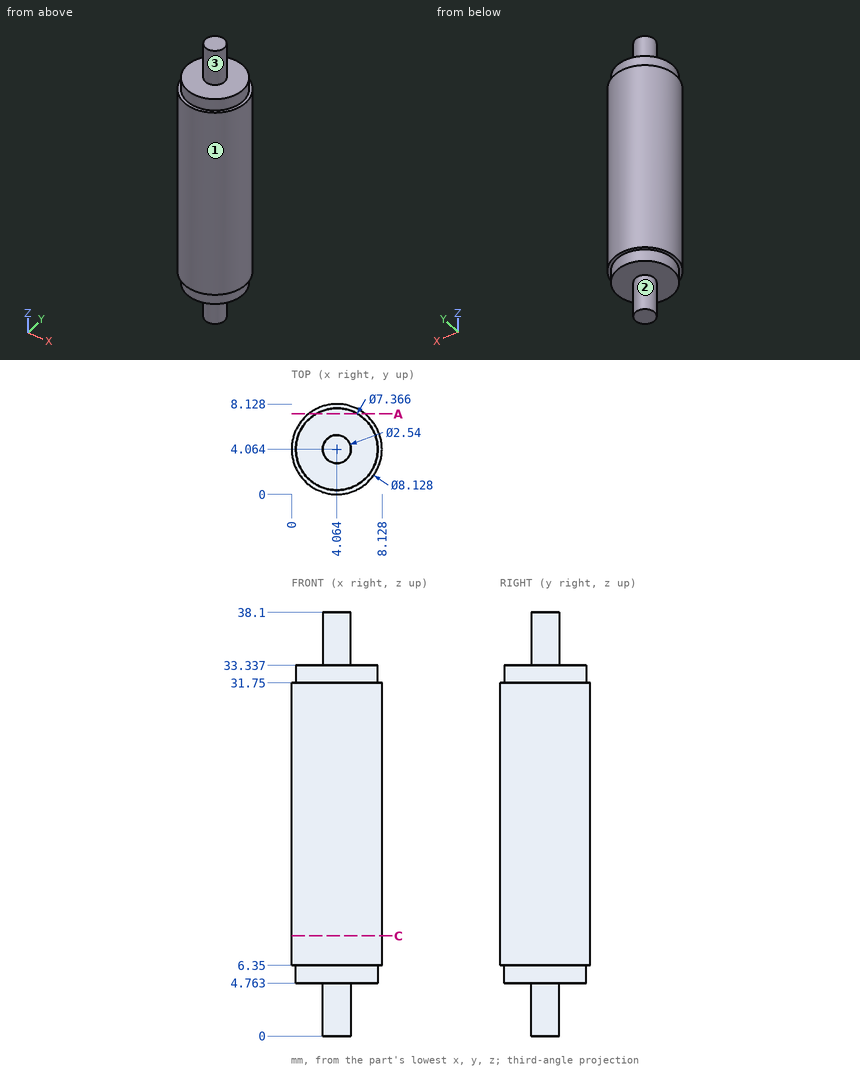
Input: dimensioned drawing with shaded views. Units: mm. Origin: part minimum x, y, z. A direction names the side the tool comes from. Give positions to 0.01 mm unless a question says otherwise; leave off trailing zeros. Order: outer loops, then holes, each group sorted by start corner. A loop starts at its lowest first (then second) coordinate and runs counter-clockwise, first axis right, second up.
(1) Access query for the marked faces 1, 2 and 3. Directions: +Z, -Z, +X, -X, +Y, -Y. A direction counts if a zero-diameter tool reaches every point of the face in a straight line with its end or side. Return the directions, or none.
(2) Contact query for flat-ended pins moving along their axis: P1, Ø1.5, axis at x = 5, z = 25.5, coming from the -Y side; P2, Ø3, axis at x = 4, y = 1, coming from the +Z side; P3, Ø1.5, axis at y = 3, z = 31, coming from the +X side. Output: stop coordinate, or through.
(3) Section query A-A (y = 7.25). Return the cut outline in (x, z), plus the area to 3 significant figures.
(4) Section query C-C (z = 9). Return the cut outline in (x, y) (1 decimal).
(5) Material intervals for line 1 along Z through (x, y) = (7.25, 1.75); line 2 along Z through (x, y) = (2.75, 2.25); line 3 along X through (y, z) = (4.25, 28.5) (1 decimal), sorted ascending.
Outcome:
1. face 1: +Z, -Z
1. face 2: -Z
1. face 3: +Z
2. P1: stops at y = 0
2. P2: stops at z = 33.34
2. P3: stops at x = 8.12
3. outline: (1.54, 6.35) - (2.22, 6.35) - (2.22, 4.76) - (5.91, 4.76) - (5.91, 6.35) - (6.59, 6.35) - (6.59, 31.75) - (5.91, 31.75) - (5.91, 33.34) - (2.22, 33.34) - (2.22, 31.75) - (1.54, 31.75) - close
3. area: 140 mm2
4. outline: circle Ø8.1 at (4.1, 4.1)
5. line 1: z = 6.35 to 31.75
5. line 2: z = 4.76 to 33.34
5. line 3: x = 0 to 8.1
